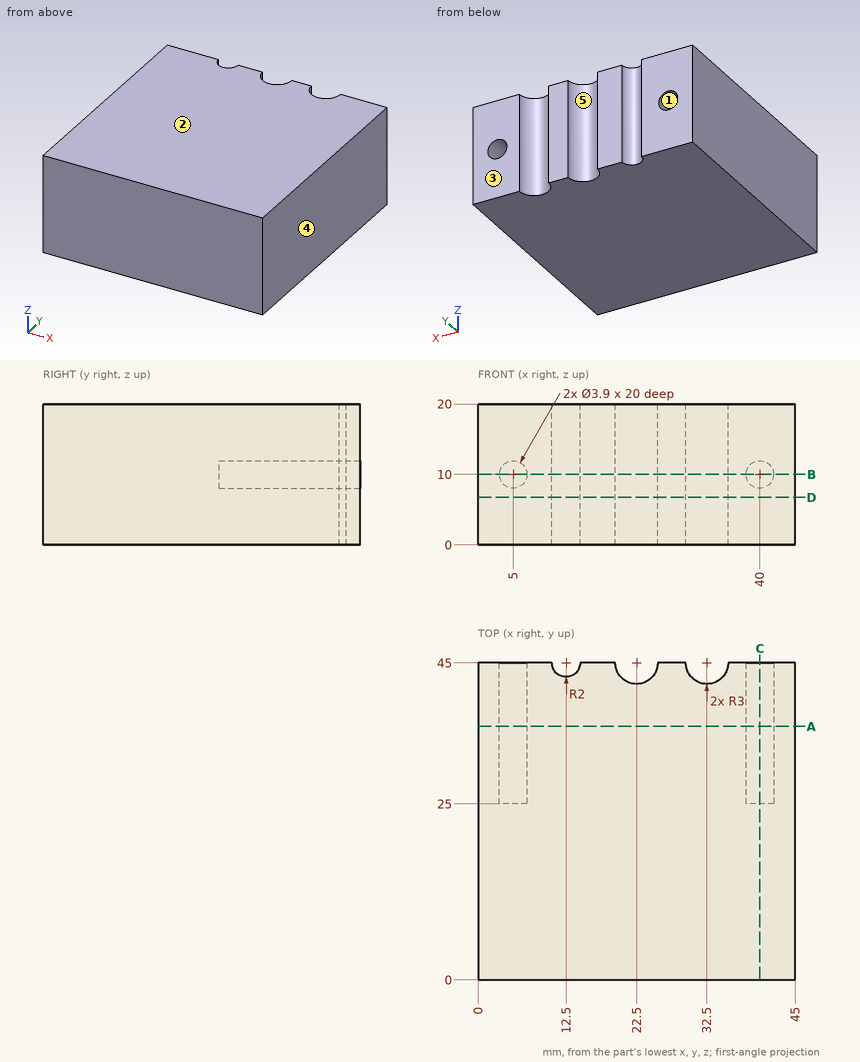
Here's the drawing with two shaded views (mm, measured from the low corner). I have some questions. A direction names the side the tool comes from. Give positions to 0.01 mm unless a question says otherwise; leave off trailing zeros. Write each loop counter-clockwise with the first axis right and the second up, starting at its lowest first coordinate (ties: lowest second). Pieces come first, ordered by that corner, then holes. Notation, with made-up numbers: (78, 12.5) - (93, 12.5) arc R13 cw to (93, 29.5) - close; hole circle Ø8 at (-40, 16). An arc over 180 degrees is marked (long way). One line per item, written item: value. Start each with the question number.
Item 1: Please list where these lines run through material, in increasing order: line 1 (X direction, y = 30, z = 10); line 2 (Z direction, x = 5, y = 32); line 3 (Y direction, x = 21, z = 6). Write a range as from..to.
Item 2: Imagine slicing it at D-D, the plane z = 6.75. List the corners of the cut face in (x, y) for me, and give its area (3 significant figures).
Item 3: Imagine slicing it at A-A, the plane y = 36. List the corners of the cut face in (x, z) for me, and give its area (3 significant figures).
Item 4: Imagine slicing it at B-B, the plane z = 10. List the corners of the cut face in (x, y) for me.
Item 5: I'm going to push flat-ended pins straight in: pin 1 (12 mm diameter, centred on y = 39.5, z = 12.5, fed in from -X); pin 2 (1.9 mm diameter, centred on x = 4.5, z = 9.5, fed in from +Y). Where does each tip first touch, or does it pass through?
Item 6: Imagine slicing it at C-C, the plane x = 40. List the corners of the cut face in (y, z) for me.
Item 7: Which directions (+Z, -Z, +X, -X, +Y, -Y) give clear straight access to the entire face, cutting with the end or side of a thin tool? Please do the marked faces 1 and 2.
Item 8: If we mould it in two halves opening along X, with no side actions, what happens to the marked faces 3, 4 and 5? For each: +X half, -X half, draft (parallel to the pull), parting line (faces both ways), or undercut.
Geometry says:
1. line 1: 0..3.05, 6.95..38.05, 41.95..45
1. line 2: 0..8.05, 11.95..20
1. line 3: 0..42.4
2. outline: (0, 0) - (45, 0) - (45, 45) - (35.5, 45) arc R3 cw to (29.5, 45) - (25.5, 45) arc R3 cw to (19.5, 45) - (14.5, 45) arc R2 cw to (10.5, 45) - (0, 45) - close
2. area: 1,990 mm^2
3. outline: (0, 0) - (45, 0) - (45, 20) - (0, 20) - close; hole circle Ø3.9 at (5, 10); hole circle Ø3.9 at (40, 10)
3. area: 876 mm^2
4. outline: (0, 0) - (45, 0) - (45, 45) - (41.95, 45) - (41.95, 25) - (38.05, 25) - (38.05, 45) - (35.5, 45) arc R3 cw to (29.5, 45) - (25.5, 45) arc R3 cw to (19.5, 45) - (14.5, 45) arc R2 cw to (10.5, 45) - (6.95, 45) - (6.95, 25) - (3.05, 25) - (3.05, 45) - (0, 45) - close
5. pin 1: x = 0
5. pin 2: y = 25
6. outline: (0, 0) - (45, 0) - (45, 8.05) - (25, 8.05) - (25, 11.95) - (45, 11.95) - (45, 20) - (0, 20) - close
7. face 1: +Y
7. face 2: +Z, +X, -X, +Y, -Y
8. face 3: draft
8. face 4: +X half
8. face 5: undercut
